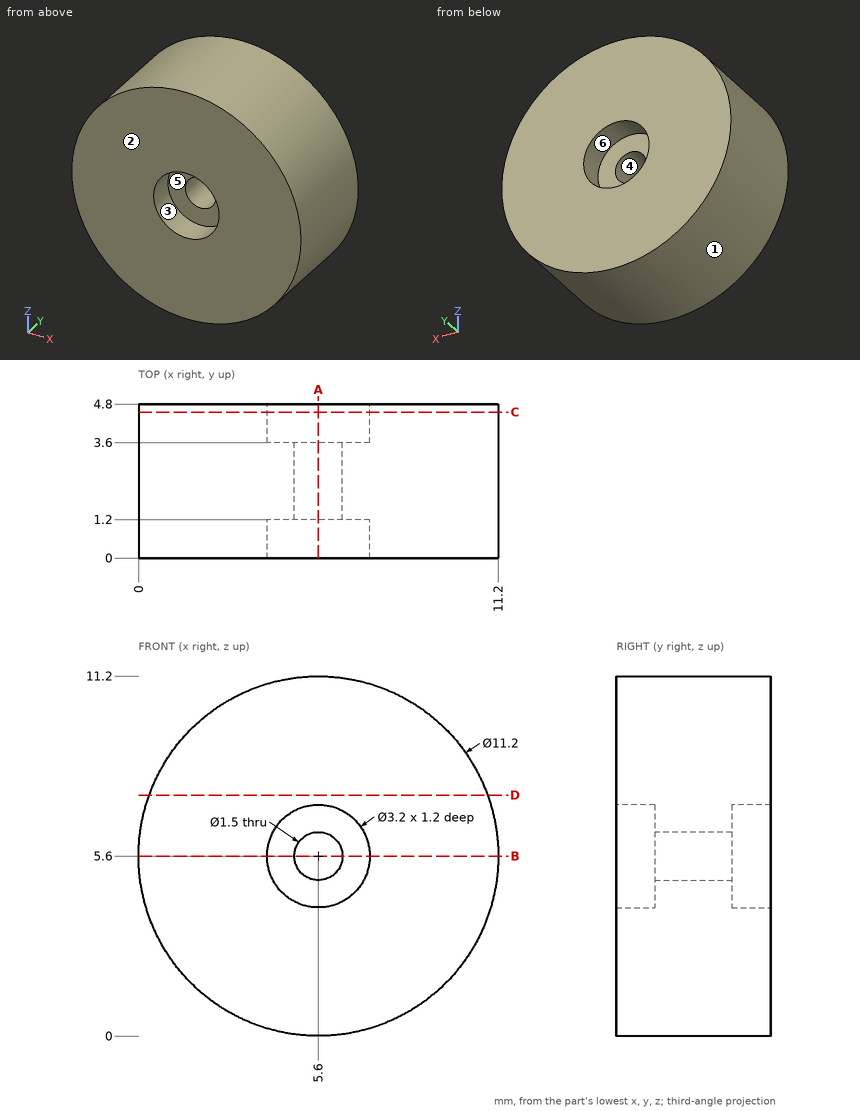
Verification items for this drawing (mm, ordinates from the low corner). A direction names the side the tool comes from. Coordinates: 2 decimals unless noted, no trailing zeros. Write each loop counter-clockwise with the first axis right and the second up, starting at its lowest first coordinate (ties: lowest second). Pieces come first, ordered by that corner, then holes. Notation, with made-up numbers: M 9,-35.5 L 59,-35.5 A19 ccw 59,-0.5 Z; hole C 2,39.5 d5. An arc over 180 degrees is marked long. One line per item, written item: value. Start each with the question number.
(1) Release check for a two-part mould opening along X. For the marked faces 1, 2 and 3 record: released by +X, released by -X, zero draft, split by the parting line, or undercut.
(2) Scan lines: line 1 along X through (y, z) = (4.5, 5.6); line 2 along X through (y, z) = (3, 5.6); line 3 along Y through (x, z) = (6, 4.5). Record each from-to range of solid material in increasing order. Write a range as [from, to].
(3) Sectioned sample at D-D, the plane z = 7.5. Enter the section's corners in (x, y), and give its area (3 significant figures).
(4) Sectioned sample at A-A, the plane x = 5.6. Enter the section's corners in (y, z).
(5) Sectioned sample at B-B, the plane z = 5.6. Enter the section's corners in (x, y).
(6) Sectioned sample at C-C, the plane y = 4.55. Enter the section's corners in (x, z).
(7) Tool access check on the marked faces 4, 5 and 6. Record the directions out of +Z, -Z, +X, -X, +Y, -Y that give a thin tool (end or side, any length) a straight path to the whole face; none if there is none.
(8) Depth check by flat-ended pin: pin 1 (1.4 mm diameter, centred on x = 5.6, z = 5.6, fed in from +Y); pin 2 (1.6 mm diameter, centred on x = 5, z = 6, fed in from +Y); pin 3 (1 mm diameter, centred on y = 1.5, z = 9, fed in from -X); pin 4 (1.6 mm diameter, centred on x = 6, z = 5, fed in from -Y). Enter the tip coordinate at first touch or a pass-through.
Filled sheet:
1. face 1: split by the parting line
1. face 2: zero draft
1. face 3: undercut
2. line 1: [0, 4], [7.2, 11.2]
2. line 2: [0, 4.85], [6.35, 11.2]
2. line 3: [1.2, 3.6]
3. outline: M 0.33,0 L 10.87,0 L 10.87,4.8 L 0.33,4.8 Z
3. area: 50.6 mm²
4. outline: M 0,0 L 4.8,0 L 4.8,4 L 3.6,4 L 3.6,4.85 L 1.2,4.85 L 1.2,4 L 0,4 Z; M 0,7.2 L 1.2,7.2 L 1.2,6.35 L 3.6,6.35 L 3.6,7.2 L 4.8,7.2 L 4.8,11.2 L 0,11.2 Z
5. outline: M 0,0 L 4,0 L 4,1.2 L 4.85,1.2 L 4.85,3.6 L 4,3.6 L 4,4.8 L 0,4.8 Z; M 6.35,1.2 L 7.2,1.2 L 7.2,0 L 11.2,0 L 11.2,4.8 L 7.2,4.8 L 7.2,3.6 L 6.35,3.6 Z
6. outline: C 5.6,5.6 d11.2; hole C 5.6,5.6 d3.2
7. face 4: +Y, -Y
7. face 5: -Y
7. face 6: +Y
8. pin 1: through
8. pin 2: y = 3.6
8. pin 3: x = 0.81
8. pin 4: y = 1.2
